Check sheet for the modelled part. Datum: model origin and axes. Units: mm. A direction names the side the tool comes from. Give positions to 0.01 mm unless a question says otherwise; leave off trailing zeros. Order: outer loops, then holes, each group sorted by start corner. A loop starts at its lowest first (then second) coordinate and runs counter-clockwise, first axis right, second up. Notation, with made-up numbers: (17.5, 9.5) -> (75.5, 9.5) arc R16 ccw to (75.5, 18.5) -> close; hole circle Ø4 at (-25, 67.25). An arc over 180 degrees is marked (long way). Answer in a Markdown table with one row per item. Add a question column.
(1) Release check for a two-part mould opening along X. For faces 5 (the face through (-8, 3, 15)), 6 (the face through (-8.5, 3, 0)), 7 (the face through (12.419, 0.507, -14.426)), 8 (the face through (16.5, 0.5, 0.2)) record: released by +X, released by -X, zero draft, split by the parting line, or undercut.
(2) Go/stop test with flat-tipped pins: pin 1 (5 mm diameter, centred on x = 4, z = -2.5, fed in from +Y); pin 2 (1.5 mm diameter, centred on y = 2.5, z = 4, fed in from -X); pin 3 (0.8 mm diameter, centred on x = 8, y = 3, fed in from +Z); pin 4 (2.5 mm diameter, centred on x = -12.9, z = 12.9, fed in from +Y). Record where each tip stops, or that it passes through.
(3) Thickness scan on L1, parallel to X at y = 0.25, z = 12.9; L2, parallel to X at y = 3.3, z = -9; L3, parallel to Y at x = 10, z = 14. Record the ranges inside material, lowest first. Write a range as [from, to].
(4) Cross-section at D-D (z = 12.9). Record the cut outline in (x, y).
(5) Cross-section at A-A (y = 2.6). Record the cut outline in (x, z), then the cut area to 3 significant figures.
(6) Cross-section at B-B (z = 0). Record the cut outline in (x, y).
(7) Set-up check for faces 1 (the face through (-7.5, 3, 0)), 2 (the face through (-8, 3, -15)), 3 (the face through (8, 3, 15)), 4 (the face through (8.5, 3, 0)): record each of +Z, -Z, +X, -X, +Y, -Y from which the full face is reachable in a straight line by a thin tool's end or side.
(8) Cross-section at C-C (x = 0). Record the cut outline in (y, z), then the cut area to 3 significant figures.
```python
from build123d import *

# Parameters (mm, degrees)
SKETCH_1_W          = 33
SKETCH_1_H          = 33
EXTRUDE_1_DEPTH     = 1
SKETCH_2_R          = 6.1
SKETCH_2_R_2        = 1.6
CUT_EXTRUDE_1_DEPTH = 24.355941428
SKETCH_3_W          = 1
SKETCH_3_H          = 30
EXTRUDE_2_DEPTH     = 5


with BuildPart() as part:
    # 草图1 → 凸台-拉伸1 (new body)
    with BuildSketch(Plane(origin=(0, 0, 0), x_dir=(1, 0, 0), z_dir=(0, 1, 0))):
        Rectangle(SKETCH_1_W, SKETCH_1_H)
    extrude(amount=EXTRUDE_1_DEPTH)

    # 草图2 → 切除-拉伸1 (cut, through all)
    with BuildSketch(Plane(origin=(0, 1, 0), x_dir=(1, 0, 0), z_dir=(0, 1, 0))):
        with Locations(Location((0, 0, 0), (0, 0, 270))):
            Circle(SKETCH_2_R)
        with Locations(Location((-12.9, 12.9, 0), (0, 0, 270))):
            Circle(SKETCH_2_R_2)
        with Locations(Location((12.9, 12.9, 0), (0, 0, 90))):
            Circle(SKETCH_2_R_2)
        with Locations(Location((12.9, -12.9, 0), (0, 0, 270))):
            Circle(SKETCH_2_R_2)
        with Locations(Location((-12.9, -12.9, 0), (0, 0, 90))):
            Circle(SKETCH_2_R_2)
    extrude(amount=-CUT_EXTRUDE_1_DEPTH, mode=Mode.SUBTRACT)

    # 草图3 → 凸台-拉伸2 (add)
    with BuildSketch(Plane(origin=(0, 1, 0), x_dir=(1, 0, 0), z_dir=(0, 1, 0))):
        with Locations((-8, 0)):
            Rectangle(SKETCH_3_W, SKETCH_3_H)
        with Locations((8, 0)):
            Rectangle(SKETCH_3_W, SKETCH_3_H)
    extrude(amount=EXTRUDE_2_DEPTH)


solid = part.part
```
Answer below:
| question | item | result |
|---|---|---|
| 1 | face 5 | zero draft |
| 1 | face 6 | released by -X |
| 1 | face 7 | undercut |
| 1 | face 8 | released by +X |
| 2 | pin 1 | stops at y = 1 |
| 2 | pin 2 | stops at x = -8.5 |
| 2 | pin 3 | stops at z = 15 |
| 2 | pin 4 | passes through |
| 3 | L1 | x = [-16.5, -14.5], [-11.3, 11.3], [14.5, 16.5] |
| 3 | L2 | x = [-8.5, -7.5], [7.5, 8.5] |
| 3 | L3 | y = [0, 1] |
| 4 | outline | (-16.5, 0) -> (-14.5, 0) -> (-14.5, 1) -> (-16.5, 1) -> close; (-11.3, 0) -> (11.3, 0) -> (11.3, 1) -> (8.5, 1) -> (8.5, 6) -> (7.5, 6) -> (7.5, 1) -> (-7.5, 1) -> (-7.5, 6) -> (-8.5, 6) -> (-8.5, 1) -> (-11.3, 1) -> close; (14.5, 0) -> (16.5, 0) -> (16.5, 1) -> (14.5, 1) -> close |
| 5 | outline | (-8.5, -15) -> (-7.5, -15) -> (-7.5, 15) -> (-8.5, 15) -> close; (7.5, -15) -> (8.5, -15) -> (8.5, 15) -> (7.5, 15) -> close |
| 5 | area | 60.0 mm² |
| 6 | outline | (-16.5, 0) -> (-6.1, 0) -> (-6.1, 1) -> (-7.5, 1) -> (-7.5, 6) -> (-8.5, 6) -> (-8.5, 1) -> (-16.5, 1) -> close; (6.1, 0) -> (16.5, 0) -> (16.5, 1) -> (8.5, 1) -> (8.5, 6) -> (7.5, 6) -> (7.5, 1) -> (6.1, 1) -> close |
| 7 | face 1 | +Z, -Z, +Y |
| 7 | face 2 | -Z, +X, -X, +Y |
| 7 | face 3 | +Z, +X, -X, +Y |
| 7 | face 4 | +Z, -Z, +X, +Y |
| 8 | outline | (0, -16.5) -> (1, -16.5) -> (1, -6.1) -> (0, -6.1) -> close; (0, 6.1) -> (1, 6.1) -> (1, 16.5) -> (0, 16.5) -> close |
| 8 | area | 20.8 mm² |
